Autodesk Inventor part; units mm, degrees
ref_plane "YZ Plane" through (0, 0, 0) normal (1, 0, 0) x (0, 1, 0)
ref_plane "XZ Plane" through (0, 0, 0) normal (0, 1, 0) x (-1, 0, 0)
ref_plane "XY Plane" through (0, 0, 0) normal (0, 0, 1) x (1, 0, 0)
sketch "Sketch1" plane through (0, 0, 0) normal (0, 0, 1) x (1, 0, 0)
  line L0 (0, 0) -> (190.5, 0)
  line L1 (190.5, 0) -> (190.5, 25.4)
  line L2 (190.5, 25.4) -> (0, 25.4)
  line L3 (0, 25.4) -> (0, 0)
  line L4 (0, 12.7) -> (190.5, 12.7) construction
  circle A0 centre (95.25, 12.7) radius 11
  line L5 (0, 0) -> (25.4, 25.4)
  circle A1 centre (177.8, 15.875) radius 25.4 construction
  circle A2 centre (177.8, 15.875) radius 1.7526
  circle A3 centre (44.45, 9.525) radius 1.7526
  dimension "d0" = 190.5
  dimension "d1" = 25.4
  dimension "d6" = 22
  dimension "d7" = 95.25
  dimension "d8" = 45
  dimension "d9" = 50.8
  dimension "d10" = 3.5052
  dimension "d11" = 12.7
  dimension "d12" = 9.525
  dimension "d13" = 3.5052
  dimension "d14" = 9.525
  dimension "d15" = 44.45
extrude "Extrusion1" add sketch "Sketch1" along normal blind 6.35 contours L5 L2 L1 L0
properties part number "Side_Plate" material "UHMW, White"
Read the model definition and answer for the solid it produces. Units are mm, in the model's axes. Coordinates: 2 decimals unless noted, no trailing zeros. Write each loop counter-clockwise with the first axis right and the second up, starting at its lowest first coordinate (ties: lowest second). Pieces come first, ordered by that corner, then holes. Notation, with made-up numbers: (89.5, -24.75) - (131.5, -24.75) arc R20 cw to (131.5, -10.75) - close; hole circle Ø3 at (17.5, -13.75). An arc over 180 degrees is marked (long way). Answer as a JSON object with one key per item and string values. Group by question number.
1. The mould has two halves that part along X. Classify faces 1 (the cylindrical face through (84.26, 12.22, 3.13)), 2 (the flat face through (109, 25.4, 3)), 3 (the cylindrical face through (176.05, 15.8, 3.13)), 4 (the flat face through (13, 13, 3)): +X half, -X half, draft (parallel to the pull), parting line (faces both ways), or undercut.
2. Consider L1, parallel to Y at x = 177.8, z = 4; L2, parallel to X at y = 14.5, z = 4.5; L3, parallel to Y at x = 44.45, z = 4.5. Determine where each line is inside the solid, lowest interval first. Write a range as [from, to].
3. A cutting plane is placed at D-D (x = 22). Determine the outline of the cut face in (y, z).
4. A cutting plane is placed at C-C (z = 5.25). Determine the outline of the cut face in (x, y) (3 decimals), plus the area to 3 significant figures.
5. A cutting plane is placed at A-A (x = 177.8). Determine the outline of the cut face in (y, z), plus the area to 3 significant figures.
6. This flat-tipped pin is pushed along its axis until it touches: P1, Ø2, axis at x = 44.45, y = 9.525, coming from the -Z side. Where does it stop, or does it pass through?
7. A cutting plane is placed at B-B (y = 20). Determine the outline of the cut face in (x, z), plus the area to 3 significant figures.
Worked out:
{
 "1": {"face 1": "undercut", "face 2": "draft", "face 3": "undercut", "face 4": "-X half"},
 "2": {"L1": "y = [0, 14.12], [17.63, 25.4]", "L2": "x = [14.5, 84.4], [106.1, 176.71], [178.89, 190.5]", "L3": "y = [0, 7.77], [11.28, 25.4]"},
 "3": {"outline": "(0, 0) - (22, 0) - (22, 6.35) - (0, 6.35) - close"},
 "4": {"outline": "(0, 0) - (190.5, 0) - (190.5, 25.4) - (25.4, 25.4) - close; hole circle Ø3.505 at (44.45, 9.525); hole circle Ø22 at (95.25, 12.7); hole circle Ø3.505 at (177.8, 15.875)", "area": "4,120 mm²"},
 "5": {"outline": "(0, 0) - (14.12, 0) - (14.12, 6.35) - (0, 6.35) - close; (17.63, 0) - (25.4, 0) - (25.4, 6.35) - (17.63, 6.35) - close", "area": "139 mm²"},
 "6": {"P1": "passes through"},
 "7": {"outline": "(20, 0) - (87.02, 0) - (87.02, 6.35) - (20, 6.35) - close; (103.48, 0) - (190.5, 0) - (190.5, 6.35) - (103.48, 6.35) - close", "area": "978 mm²"}
}
